```python
from build123d import *

# Parameters (mm, degrees)
SKETCH1_W           = 200
SKETCH1_H           = 98
SKETCH1_R           = 4
BOSS_EXTRUDE1_DEPTH = 3


with BuildPart() as part:
    # Sketch1 → Boss-Extrude1 (new body)
    with BuildSketch(Plane.XY):
        with Locations((-26.405797101, 15.623188406)):
            Rectangle(SKETCH1_W, SKETCH1_H)
        with Locations((47.680210455, 51.925332109)):
            Circle(SKETCH1_R, mode=Mode.SUBTRACT)
        with Locations(Location((-100.491804658, 51.925332109, 0), (0, 0, 180))):
            Circle(SKETCH1_R, mode=Mode.SUBTRACT)
        with Locations((-100.491804658, -20.678955297)):
            Circle(SKETCH1_R, mode=Mode.SUBTRACT)
        with Locations(Location((47.680210455, -20.678955297, 0), (0, 0, 180))):
            Circle(SKETCH1_R, mode=Mode.SUBTRACT)
        with Locations((-100.491804658, 15.623188406)):
            Circle(SKETCH1_R, mode=Mode.SUBTRACT)
        with Locations(Location((47.680210455, 15.623188406, 0), (0, 0, 180))):
            Circle(SKETCH1_R, mode=Mode.SUBTRACT)
        with Locations((-26.405797101, 51.925332109)):
            Circle(SKETCH1_R, mode=Mode.SUBTRACT)
        with Locations(Location((-26.405797101, -20.678955297, 0), (0, 0, 180))):
            Circle(SKETCH1_R, mode=Mode.SUBTRACT)
    extrude(amount=BOSS_EXTRUDE1_DEPTH)


solid = part.part
```
Check sheet for the modelled part. Datum: model origin and axes. Units: mm. Round coordinates to 2 decimals unless told otherwise and drop trailing zeros. Loops run counter-clockwise (first coordinate to the right, second up) from the corner with the lowest first, then second, coordinate; pieces in that order, holes last. Notation, with made-up numbers: (55, -10) - (79, -10) arc R20 cw to (79, 11) - close; hole circle Ø10 at (-37, -13.5). An arc over 180 degrees is marked (long way). Write item = value, one per line. Start each with the question number.
Q1. Release check for a two-part mould opening along Y. For faces 1 (the face through (-96.677, -19.477, 1.479)), 2 (the face through (-28, 16, 0)) record: pulls with the +Y half, pulls with the -Y half, needs draft (parallel to the pull), parting line crosses it, or undercut.
Q2. Section check A-A (x = -101.5). Record the boundary of the cut face in (y, z), plus the area to 3 significant figures.
Q3. Section check B-B (z = 2.4). Count the separate pieces of the cut face and the enclosed holes in it, plus the area to 3 significant figures.
Q4. Thickness scan on L1, parallel to X at y = 15.5, z = 0.5; L2, parallel to X at y = -22, z = 1.65; L3, parallel to X at y = 18, z = 2.15. Record the ranges inside material, lowest first.
Q5. Section check D-D (x = 47.5). Record the boundary of the cut face in (y, z), plus the area to 3 significant figures.
Q6. Section check C-C (x = -25). Record the boundary of the cut face in (y, z).
Derived:
q1.face_1 = undercut
q1.face_2 = needs draft
q2.outline = (-33.38, 0) - (-24.55, 0) - (-24.55, 3) - (-33.38, 3) - close; (-16.81, 0) - (11.75, 0) - (11.75, 3) - (-16.81, 3) - close; (19.49, 0) - (48.05, 0) - (48.05, 3) - (19.49, 3) - close; (55.8, 0) - (64.62, 0) - (64.62, 3) - (55.8, 3) - close
q2.area = 224 mm^2
q3.separate_pieces = 1
q3.enclosed_holes = 8
q3.area = 19,200 mm^2
q4.L1 = -126.41 to -104.49, -96.49 to 43.68, 51.68 to 73.59
q4.L2 = -126.41 to -104.27, -96.72 to -30.18, -22.63 to 43.9, 51.46 to 73.59
q4.L3 = -126.41 to -103.71, -97.27 to 44.46, 50.9 to 73.59
q5.outline = (-33.38, 0) - (-24.67, 0) - (-24.67, 3) - (-33.38, 3) - close; (-16.68, 0) - (11.63, 0) - (11.63, 3) - (-16.68, 3) - close; (19.62, 0) - (47.93, 0) - (47.93, 3) - (19.62, 3) - close; (55.92, 0) - (64.62, 0) - (64.62, 3) - (55.92, 3) - close
q5.area = 222 mm^2
q6.outline = (-33.38, 0) - (-24.42, 0) - (-24.42, 3) - (-33.38, 3) - close; (-16.93, 0) - (48.18, 0) - (48.18, 3) - (-16.93, 3) - close; (55.67, 0) - (64.62, 0) - (64.62, 3) - (55.67, 3) - close
